Autodesk Inventor part; units mm, degrees
ref_plane "YZ Plane" through (0, 0, 0) normal (1, 0, 0) x (0, 1, 0)
ref_plane "XZ Plane" through (0, 0, 0) normal (0, 1, 0) x (-1, 0, 0)
ref_plane "XY Plane" through (0, 0, 0) normal (0, 0, 1) x (1, 0, 0)
sketch "Skizze1" plane through (0, 0, 0) normal (0, 0, 1) x (1, 0, 0)
  line L0 (-32.5, 32.5) -> (32.5, 32.5)
  line L1 (32.5, 32.5) -> (32.5, -32.5)
  line L2 (32.5, -32.5) -> (-32.5, -32.5)
  line L3 (-32.5, -32.5) -> (-32.5, 32.5)
  point P0 (0, 0)
  point P1 (-32.5, 16.5982)
  point P2 (-16.4712, 32.5)
  dimension "d0" = 65
  dimension "d1" = 65
  dimension "d2" = 32.5
  dimension "d3" = 32.5
extrude "Extrusion1" add sketch "Skizze1" along normal blind 100
sketch "Skizze2" plane through (0, 0, 100) normal (0, 0, 1) x (1, 0, 0)
  circle A0 centre (0, 0) radius 10
  dimension "d6" = 20
extrude "Extrusion2" add sketch "Skizze2" along normal blind 2
sketch "Skizze3" plane through (0, 0, 102) normal (0, 0, 1) x (1, 0, 0)
  circle A0 centre (0, 0) radius 4
  dimension "d9" = 8
extrude "Extrusion3" add sketch "Skizze3" along normal blind 15
sketch "Sketch4" plane through (0, 0, 100) normal (0, 0, 1) x (1, 0, 0)
  line L0 (32.5, 32.5) -> (-32.5, 32.5)
  line L1 (-14.5, 32.5) -> (-32.5, 22.9292)
  line L2 (-32.5, 32.5) -> (-32.5, -32.5)
  line L3 (-32.5, 32.5) -> (-14.5, 32.5)
  line L4 (-32.5, 32.5) -> (-32.5, 22.9292)
  point P0 (0, 0)
  dimension "d15" = 28
  dimension "d16" = 18
extrude "Extrusion4" cut sketch "Sketch4" against normal up to surface (100 mm away)
mirror "Mirror1" about plane through (0, 0, 0) normal (1, 0, 0) of "Extrusion4"
mirror "Mirror2" about plane through (0, 0, 0) normal (0, 1, 0) of "Extrusion4", "Mirror1"
sketch "Sketch5" plane through (0, 0, 0) normal (1, 0, 0) x (0, 1, 0)
  line L0 (32.5, 0) -> (32.5, 100)
  line L1 (32.5, 20.5) -> (36.5, 20.5)
  line L2 (36.5, 20.5) -> (36.5, 22.5)
  line L3 (36.5, 22.5) -> (40.3063, 22.5)
  line L4 (47.5, 30) -> (32.5, 30)
  line L5 (32.5, 20.5) -> (32.5, 30)
  line L6 (22.9292, 0) -> (32.5, 0)
  arc A0 (40.3063, 22.5) -> (47.5, 27) centre (40.3063, 30.5) ccw
  line L7 (47.5, 27) -> (47.5, 30)
  point P0 (0, 0)
  dimension "d19" = 4
  dimension "d20" = 2
  dimension "d21" = 15
  dimension "d22" = 30
  dimension "d23" = 15
  dimension "d24" = 8
  dimension "d25" = 3
revolve "Revolution1" add sketch "Sketch5" angle 360 about axis through (0, 47.5, 30) along (0, -1, 0)
equation "\"d1\" = d0"
properties part number "motor" material "Stahl"
Design review of the part built by this model. Coordinates are the model's own, in mm. A direction names the side the tool comes from. Give positions to 0.01 mm unless a question says otherwise; leave off trailing zeros. Write each loop counter-clockwise with the first axis right and the second up, starting at its lowest first coordinate (ties: lowest second). Pieces come first, ordered by that corner, then holes. Notation, with made-up numbers: (-2.5, 45) -> (38.5, 45) arc R27 cw to (38.5, 81) -> close; hole circle Ø6 at (-2, 56.25). An arc over 180 degrees is marked (long way). Answer in a Markdown table with one row per item.
(1) Consider section C-C (x = -27.5). State the section outline as (y, z) points.
Results:
| item | result |
|---|---|
| outline | (-25.59, 0) -> (25.59, 0) -> (25.59, 100) -> (-25.59, 100) -> close |
(2) For faces 1 (the cylindrical face through (5.78, 34.53, 37.54)), 2 (the flat face through (4.3, 0.1, 102)), 3 (the flat face through (0, 47.5, 30)), list the 3-axis set-ups (+Z, -Z, +X, -X, +Y, -Y) from which the entire face can be reached by the end or side of a thin tool; tool diameter is ignored.
Results:
| item | result |
|---|---|
| face 1 | +Y |
| face 2 | +Z |
| face 3 | +Z, -Z, +X, -X, +Y |
(3) To check wall thickness, follow probe 1 along Z at (x, y) = (-21, 12.5); probe 2 along Y at (x, z) = (-5, 68); probe 3 along Z at (x, y) = (-9.5, -2.5). State the ranges of each line that lie inside material, in increasing order.
Results:
| item | result |
|---|---|
| probe 1 | 0 to 100 |
| probe 2 | -32.5 to 32.5 |
| probe 3 | 0 to 102 |
(4) Consider section A-A (z = 48). State the section outline as (x, y) points.
Results:
| item | result |
|---|---|
| outline | (-32.5, -22.93) -> (-14.5, -32.5) -> (14.5, -32.5) -> (32.5, -22.93) -> (32.5, 22.93) -> (14.5, 32.5) -> (-14.5, 32.5) -> (-32.5, 22.93) -> close |
(5) Consider section B-B (y = -2). State the section outline as (x, z) points, then the cut area to 3 significant figures.
Results:
| item | result |
|---|---|
| outline | (-32.5, 0) -> (32.5, 0) -> (32.5, 100) -> (9.8, 100) -> (9.8, 102) -> (3.46, 102) -> (3.46, 117) -> (-3.46, 117) -> (-3.46, 102) -> (-9.8, 102) -> (-9.8, 100) -> (-32.5, 100) -> close |
| area | 6,640 mm2 |
(6) Consider section D-D (y = 25.5). State the section outline as (x, z) points, then the cut area to 3 significant figures.
Results:
| item | result |
|---|---|
| outline | (-27.67, 0) -> (27.67, 0) -> (27.67, 100) -> (-27.67, 100) -> close |
| area | 5,530 mm2 |
(7) Clearance check with flat-ended pins moving along their axes: pin 1 (1 mm diameter, centred on x = 22, z = 24.5, fed in from +Y); pin 2 (1.5 mm diameter, centred on x = 16.5, z = 29.5, fed in from -Y); pin 3 (10 mm diameter, centred on x = -25.5, y = -8, fed in from +Z). State where each tip first meets the part, or that it passes through.
Results:
| item | result |
|---|---|
| pin 1 | y = 28.78 |
| pin 2 | y = -31.84 |
| pin 3 | z = 100 |
